```python
from build123d import *

# Parameters (mm, degrees)
BOSS_EXTRUDE1_DEPTH = 4
CUT_EXTRUDE1_REACH  = 70.376
SKETCH2_R           = 15
FILLET1_R           = 1
SKETCH4_R           = 25
SKETCH4_R_2         = 15
CUT_EXTRUDE2_DEPTH  = 2.4


with BuildPart() as part:
    # Sketch1 → Boss-Extrude1 (new body)
    with BuildSketch(Plane(origin=(0, 0, 0), x_dir=(1, 0, 0), z_dir=(0, 1, 0))):
        Polygon((-41, 38), (-41, 45), (41, 45), (41, 38), (47, 38), (47, -38), (41, -38), (41, -49.5), (-41, -49.5), (-41, -38), (-47, -38), (-47, 38), align=None)
    extrude(amount=BOSS_EXTRUDE1_DEPTH)

    # Sketch2 → Cut-Extrude1 (cut, up to next)
    with BuildSketch(Plane(origin=(0, 4, 0), x_dir=(1, 0, 0), z_dir=(0, 1, 0)), mode=Mode.PRIVATE) as cut_extrude1_sk1:
        with Locations(Location((0, 0, 0), (0, 0, 270))):
            Circle(SKETCH2_R)
    cut_extrude1_tool1 = extrude(cut_extrude1_sk1.sketch, amount=-CUT_EXTRUDE1_REACH, mode=Mode.PRIVATE) & part.part
    add(cut_extrude1_tool1.solids().sort_by_distance((0, 4, 0))[0], mode=Mode.SUBTRACT)

    # Fillet1
    fillet1_edges = [part.edges().sort_by_distance(p)[0] for p in [
        (41, 2, 38),
        (-41, 2, 38),
        (-41, 2, -38),
        (41, 2, -38),
    ]]
    fillet(fillet1_edges, radius=FILLET1_R)

    # Sketch4 → Cut-Extrude2 (cut)
    with BuildSketch(Plane(origin=(0, 4, 0), x_dir=(1, 0, 0), z_dir=(0, 1, 0))):
        with Locations(Location((0, 0, 0), (0, 0, 270))):
            Circle(SKETCH4_R)
        with Locations(Location((0, 0, 0), (0, 0, 270))):
            Circle(SKETCH4_R_2, mode=Mode.SUBTRACT)
    extrude(amount=-CUT_EXTRUDE2_DEPTH, mode=Mode.SUBTRACT)


solid = part.part
```
Could you check a few things on this model? Use its own coordinates, in mm. A direction names the side the tool comes from. Coordinates: 2 decimals unless noted, no trailing zeros. Loops run counter-clockwise (first coordinate to the right, second up) from the corner with the lowest first, then second, coordinate; pieces in that order, holes last. Notation, with made-up numbers: M 39.25,17.25 L 58.25,17.25 A30 cw 58.25,41.25 Z; hole C 67,-3 d1. An arc over 180 degrees is marked long. Put each result on its own line as item: value. Start each with the question number.
(1) Suppose I cut it at B-B on y = 3.3. Please give me the cut outline in (x, z).
(2) I need wall thicknesses on line 1 (X direction, y = 3.1, z = 0); line 2 (X direction, y = 1, z = 0); line 3 (Y direction, x = -14, z = 10). Which ranges of each line are inside material? Lowest first, please. Write a range as from..to.
(3) Will these pins go through, and if not, where does the flat tip stop? P1, Ø1.2, axis at x = 44.5, y = 2.5, coming from the +Z side; P2, Ø2, axis at y = 1.5, z = -40.5, coming from the -X side.
(4) Suppose I cut it at C-C on z = 0. Please give me the cut outline in (x, y), then the cut area to 3 significant figures.
(5) Suppose I cut it at A-A on x = 0. Please give me the cut outline in (y, z).
(6) Suppose I cut it at D-D on z = 23.5. Please give me the cut outline in (x, y).
(7) For faces 4 (the face through (7.509, 2.817, 23.846)), 5 (the face through (45, 2, 38)), 6 (the face through (44, 2, -38)), which set-ups out of +Z, -Z, +X, -X, +Y, -Y let a thin tool reach every point of the face, with its end or its side?
(8) Thinking about a two-plate mould opening in Z: for faces 1 (the face through (-44, 2, 38)), 2 (the face through (-11, 1.6, 11)), 3 (the face through (-41, 2, 44)), which applies, pulls with the +Z half, pulls with the -Z half, needs draft (parallel to the pull), parting line crosses it, or undercut?
Solutions:
1. outline: M -47,-38 L -42,-38 A1 cw -41,-39 L -41,-45 L 41,-45 L 41,-39 A1 cw 42,-38 L 47,-38 L 47,38 L 42,38 A1 cw 41,39 L 41,49.5 L -41,49.5 L -41,39 A1 cw -42,38 L -47,38 Z; hole C 0,0 d50
2. line 1: x = -47..-25, 25..47
2. line 2: x = -47..-15, 15..47
2. line 3: y = 0..1.6
3. P1: stops at z = 38
3. P2: stops at x = -41
4. outline: M -47,0 L -15,0 L -15,1.6 L -25,1.6 L -25,4 L -47,4 Z; M 15,0 L 47,0 L 47,4 L 25,4 L 25,1.6 L 15,1.6 Z
4. area: 208 mm2
5. outline: M 0,-45 L 4,-45 L 4,-25 L 1.6,-25 L 1.6,-15 L 0,-15 Z; M 0,15 L 1.6,15 L 1.6,25 L 4,25 L 4,49.5 L 0,49.5 Z
6. outline: M -47,0 L 47,0 L 47,4 L 8.53,4 L 8.53,1.6 L -8.53,1.6 L -8.53,4 L -47,4 Z
7. face 4: +Y
7. face 5: +Z, +X, +Y, -Y
7. face 6: -Z, +X, +Y, -Y
8. face 1: pulls with the +Z half
8. face 2: undercut
8. face 3: needs draft
